Autodesk Inventor part; units mm, degrees
ref_plane "YZ Plane" through (0, 0, 0) normal (1, 0, 0) x (0, 1, 0)
ref_plane "XZ Plane" through (0, 0, 0) normal (0, 1, 0) x (-1, 0, 0)
ref_plane "XY Plane" through (0, 0, 0) normal (0, 0, 1) x (1, 0, 0)
sketch "Sketch1" plane through (0, 0, 0) normal (0, 1, 0) x (-1, 0, 0)
  line L0 (0, 0) -> (12.7, 0)
  line L1 (12.7, 0) -> (12.7, 114.3)
  line L2 (12.7, 114.3) -> (0, 114.3)
  line L3 (0, 114.3) -> (0, 0)
  circle A0 centre (6.35, 6.35) radius 2.5797
  circle A1 centre (6.35, 107.95) radius 2.5797
  circle A2 centre (6.35, 6.35) radius 6.35
  circle A3 centre (6.35, 107.95) radius 6.35
  point P0 (0, 107.95)
  point P1 (0, 6.35)
  point P2 (12.7, 6.35)
  point P3 (12.7, 107.95)
  dimension "d0" = 12.7
  dimension "d2" = 6.35
  dimension "d3" = 6.35
  dimension "d4" = 5.1594
  dimension "d5" = 6.35
  dimension "d6" = 5.1594
  dimension "d7" = 6.35
  dimension "d51" = 101.6
  dimension "d52" = 12.7
  dimension "d53" = 12.7
extrude "Extrusion1" add sketch "Sketch1" along normal blind 50.8 contours A2 | L3 A3 L1 A2 | A3
sketch "Sketch5" plane through (0, 0, 107.95) normal (1, 0, 0) x (0, 0, -1)
  line L0 (107.95, 50.8) -> (101.6, 50.8)
  line L1 (0, 0) -> (107.95, 0)
  line L2 (107.95, 0) -> (107.95, 50.8)
  line L3 (107.95, 50.8) -> (0, 50.8)
  line L4 (0, 50.8) -> (0, 0)
  line L5 (107.95, 0) -> (107.95, 50.8)
  line L6 (107.95, 38.1) -> (82.55, 38.1)
  line L7 (82.55, 38.1) -> (82.55, 12.7)
  line L8 (82.55, 12.7) -> (107.95, 12.7)
  line L9 (107.95, 12.7) -> (107.95, 38.1)
  line L10 (101.6, 50.8) -> (0, 50.8)
  line L11 (-6.35, 0) -> (-6.35, 50.8)
  line L12 (0, 50.8) -> (-6.35, 50.8)
  line L13 (-6.35, 50.8) -> (-6.35, 0)
  line L14 (-6.35, 0) -> (0, 0)
  line L15 (0, 0) -> (0, 50.8)
  line L16 (-6.35, 0) -> (-6.35, 50.8)
  line L17 (-6.35, 12.7) -> (19.05, 12.7)
  line L18 (19.05, 12.7) -> (19.05, 38.1)
  line L19 (19.05, 38.1) -> (-6.35, 38.1)
  line L20 (-6.35, 38.1) -> (-6.35, 12.7)
  point P0 (95.25, 38.1)
  point P1 (107.95, 38.1)
  dimension "d47" = 25.4
  dimension "d48" = 25.4
  dimension "d49" = 12.7
extrude "Extrusion5" cut sketch "Sketch5" against normal through all contours L2 L8 L7 L6 | L19 L18 L17 L4 | L4 L17 L11 L19
fillet "Fillet3" radius 3.175 24 edges at (-12.7, 38.1, 15.875) (0, 38.1, 15.875) (-6.35, 38.1, 0) (-6.35, 12.7, 0) (-12.7, 12.7, 15.875) (0, 12.7, 15.875) (0, 25.4, 25.4) (-12.7, 25.4, 25.4) (-12.7, 0, 57.15) (-6.35, 0, 114.3) (0, 0, 57.15) (-6.35, 0, 0) (-6.35, 50.8, 114.3) (0, 50.8, 57.15) (-6.35, 50.8, 0) (-12.7, 50.8, 57.15) (0, 25.4, 88.9) (-12.7, 25.4, 88.9) (-6.35, 12.7, 114.3) (-12.7, 12.7, 98.425) (0, 12.7, 98.425) (0, 38.1, 98.425) (-12.7, 38.1, 98.425) (-6.35, 38.1, 114.3)
properties part number "swing pusher"
The model under review builds one solid part; all positions refer to its coordinate system, in mm. A direction names the side the tool comes from. Coordinates: 2 decimals unless noted, no trailing zeros. Loops run counter-clockwise (first coordinate to the right, second up) from the corner with the lowest first, then second, coordinate; pieces in that order, holes last. Notation, with made-up numbers: (49.5, 24.25) -> (99.5, 24.25) arc R17 ccw to (99.5, 51.25) -> close; hole circle Ø11 at (85.5, -6.75). An arc over 180 degrees is marked (long way). Use a Markdown table: item, result. Add a question column.
1. Add section B-B on y = 20. Write out the cut boundary in (x, z) (3 decimals), plus the area to 3 significant figures.
2. To check wall thickness, follow line 1 (Z direction, x = -6.35, y = 47.75); line 2 (Y direction, x = -8, z = 25); line 3 (X direction, y = 42, z = 6). State the ranges of each line that lie inside material, in increasing order.
3. Clearance check with flat-ended pins moving along their axes: pin 1 Ø3 at (x, y) = (-10.5, 33.5) entering from -Z; pin 2 Ø7 at (x, y) = (-5.5, 19.5) entering from +Z. State where each tip first meets the part, or that it passes through.
4. Add section C-C on x = -6.35. Give the number of separate pieces and of enclosed holes in the cut face, plus the area to 3 significant figures.
5. Draft analysis for pull direction X (two halves, no side actions). For faces 1 (the face through (-7.737, 44.361, 4.175)), 2 (the face through (-11.79, 0.95, 57.86)), 3 (the face through (-6, 0, 58)), state which applies: pulls with the +X half, pulls with the -X half, needs draft (parallel to the pull), parting line crosses it, or undercut.
6. Machinability: for faces 4 (the face through (-0.91, 39.05, 96.68)), 5 (the face through (-11.79, 39.05, 96.99)), 6 (the face through (-6, 12.7, 17)), 7 (the face through (-11.79, 11.75, 17.31)), which of the approach directions +Z, -Z, +X, -X, +Y, -Y give a long, thin tool a straight path to every point of the face, cutting with its end or side? Answer none if there is none.
7. Add section A-A on z = 10. Write out the cut boundary in (x, y) (3 decimals), plus the area to 3 significant figures.
Returned:
| question | item | result |
|---|---|---|
| 1 | outline | (-12.7, 28.575) arc R3.175 ccw to (-9.525, 25.4) -> (-3.175, 25.4) arc R3.175 ccw to (0, 28.575) -> (0, 85.725) arc R3.175 ccw to (-3.175, 88.9) -> (-9.525, 88.9) arc R3.175 ccw to (-12.7, 85.725) -> close |
| 1 | area | 798 mm² |
| 2 | line 1 | z = 0 to 3.77, 8.93 to 105.37, 110.53 to 114.3 |
| 2 | line 2 | y = 0 to 12.7, 38.1 to 50.8 |
| 2 | line 3 | x = -12.69 to -8.91, -3.79 to -0.01 |
| 3 | pin 1 | stops at z = 25.4 |
| 3 | pin 2 | stops at z = 88.9 |
| 4 | separate pieces | 5 |
| 4 | enclosed holes | 0 |
| 4 | area | 4,240 mm² |
| 5 | face 1 | undercut |
| 5 | face 2 | pulls with the -X half |
| 5 | face 3 | needs draft |
| 6 | face 4 | +Z, +X |
| 6 | face 5 | +Z, -X |
| 6 | face 6 | -Z, +X, -X |
| 6 | face 7 | -Z, -X |
| 7 | outline | (-12.7, 3.175) arc R3.175 ccw to (-9.525, 0) -> (-3.175, 0) arc R3.175 ccw to (0, 3.175) -> (0, 9.525) arc R3.175 ccw to (-3.175, 12.7) -> (-9.525, 12.7) arc R3.175 ccw to (-12.7, 9.525) -> close; (-12.7, 41.275) arc R3.175 ccw to (-9.525, 38.1) -> (-3.175, 38.1) arc R3.175 ccw to (0, 41.275) -> (0, 47.625) arc R3.175 ccw to (-3.175, 50.8) -> (-9.525, 50.8) arc R3.175 ccw to (-12.7, 47.625) -> close |
| 7 | area | 305 mm² |
